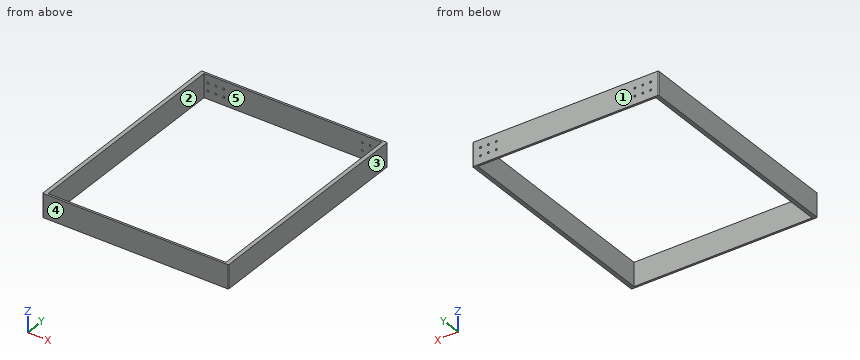
```python
from build123d import *

# Parameters (mm, degrees)
SKETCH1_W           = 599.44
SKETCH1_H           = 723.9
SKETCH1_W_2         = 574.04
SKETCH1_H_2         = 711.2
BOSS_EXTRUDE1_DEPTH = 76.2
CUT_EXTRUDE1_REACH  = 789.191
SKETCH2_R           = 3.175
FILLET1_R           = 2.54


with BuildPart() as part:
    # Sketch1 → Boss-Extrude1 (new body)
    with BuildSketch(Plane.XY):
        Rectangle(SKETCH1_W, SKETCH1_H)
        Rectangle(SKETCH1_W_2, SKETCH1_H_2, mode=Mode.SUBTRACT)
    extrude(amount=BOSS_EXTRUDE1_DEPTH)

    # Sketch2 → Cut-Extrude1 (cut, up to next)
    with BuildSketch(Plane(origin=(0, 361.95, 0), x_dir=(1, 0, 0), z_dir=(0, 1, 0)), mode=Mode.PRIVATE) as cut_extrude1_sk1:
        with Locations(Location((-274.32, -50.8, 0), (0, 0, 270))):
            Circle(SKETCH2_R)
    cut_extrude1_tool1 = extrude(cut_extrude1_sk1.sketch, amount=-CUT_EXTRUDE1_REACH, mode=Mode.PRIVATE) & part.part
    # Sketch2 → Cut-Extrude1 (cut, up to next)
    with BuildSketch(Plane(origin=(0, 361.95, 0), x_dir=(1, 0, 0), z_dir=(0, 1, 0)), mode=Mode.PRIVATE) as cut_extrude1_sk2:
        with Locations(Location((-274.32, -25.4, 0), (0, 0, 270))):
            Circle(SKETCH2_R)
    cut_extrude1_tool2 = extrude(cut_extrude1_sk2.sketch, amount=-CUT_EXTRUDE1_REACH, mode=Mode.PRIVATE) & part.part
    # Sketch2 → Cut-Extrude1 (cut, up to next)
    with BuildSketch(Plane(origin=(0, 361.95, 0), x_dir=(1, 0, 0), z_dir=(0, 1, 0)), mode=Mode.PRIVATE) as cut_extrude1_sk3:
        with Locations(Location((-248.92, -50.8, 0), (0, 0, 270))):
            Circle(SKETCH2_R)
    cut_extrude1_tool3 = extrude(cut_extrude1_sk3.sketch, amount=-CUT_EXTRUDE1_REACH, mode=Mode.PRIVATE) & part.part
    # Sketch2 → Cut-Extrude1 (cut, up to next)
    with BuildSketch(Plane(origin=(0, 361.95, 0), x_dir=(1, 0, 0), z_dir=(0, 1, 0)), mode=Mode.PRIVATE) as cut_extrude1_sk4:
        with Locations(Location((-248.92, -25.4, 0), (0, 0, 270))):
            Circle(SKETCH2_R)
    cut_extrude1_tool4 = extrude(cut_extrude1_sk4.sketch, amount=-CUT_EXTRUDE1_REACH, mode=Mode.PRIVATE) & part.part
    # Sketch2 → Cut-Extrude1 (cut, up to next)
    with BuildSketch(Plane(origin=(0, 361.95, 0), x_dir=(1, 0, 0), z_dir=(0, 1, 0)), mode=Mode.PRIVATE) as cut_extrude1_sk5:
        with Locations(Location((-223.52, -50.8, 0), (0, 0, 270))):
            Circle(SKETCH2_R)
    cut_extrude1_tool5 = extrude(cut_extrude1_sk5.sketch, amount=-CUT_EXTRUDE1_REACH, mode=Mode.PRIVATE) & part.part
    # Sketch2 → Cut-Extrude1 (cut, up to next)
    with BuildSketch(Plane(origin=(0, 361.95, 0), x_dir=(1, 0, 0), z_dir=(0, 1, 0)), mode=Mode.PRIVATE) as cut_extrude1_sk6:
        with Locations(Location((-223.52, -25.4, 0), (0, 0, 270))):
            Circle(SKETCH2_R)
    cut_extrude1_tool6 = extrude(cut_extrude1_sk6.sketch, amount=-CUT_EXTRUDE1_REACH, mode=Mode.PRIVATE) & part.part
    cut_extrude1_1 = cut_extrude1_tool1.solids().sort_by_distance((-274.32, 361.95, 50.8))[0]
    add(cut_extrude1_1, mode=Mode.SUBTRACT)
    cut_extrude1_2 = cut_extrude1_tool2.solids().sort_by_distance((-274.32, 361.95, 25.4))[0]
    add(cut_extrude1_2, mode=Mode.SUBTRACT)
    cut_extrude1_3 = cut_extrude1_tool3.solids().sort_by_distance((-248.92, 361.95, 50.8))[0]
    add(cut_extrude1_3, mode=Mode.SUBTRACT)
    cut_extrude1_4 = cut_extrude1_tool4.solids().sort_by_distance((-248.92, 361.95, 25.4))[0]
    add(cut_extrude1_4, mode=Mode.SUBTRACT)
    cut_extrude1_5 = cut_extrude1_tool5.solids().sort_by_distance((-223.52, 361.95, 50.8))[0]
    add(cut_extrude1_5, mode=Mode.SUBTRACT)
    cut_extrude1_6 = cut_extrude1_tool6.solids().sort_by_distance((-223.52, 361.95, 25.4))[0]
    add(cut_extrude1_6, mode=Mode.SUBTRACT)
    cut_extrude1 = cut_extrude1_1 + cut_extrude1_2 + cut_extrude1_3 + cut_extrude1_4 + cut_extrude1_5 + cut_extrude1_6  # Cut-Extrude1 as one shape, for the pattern or mirror that repeats it

    # Mirror1: Cut-Extrude1 across plane
    add(cut_extrude1.mirror(Plane(origin=(0, 0, 0), x_dir=(0, 0, 1), z_dir=(1, 0, 0))), mode=Mode.SUBTRACT)

    # Fillet1
    fillet1_edges = [part.edges().sort_by_distance(p)[0] for p in [
        (-299.72, -361.95, 38.1),
        (-299.72, 361.95, 38.1),
        (299.72, 361.95, 38.1),
        (299.72, -361.95, 38.1),
    ]]
    fillet(fillet1_edges, radius=FILLET1_R)


solid = part.part
```
Input: part model. Units: mm. Frame: model coordinates. Face numbers are marked on the shaded views. A direction names the side the tool comes from. Give positions to 0.01 mm unless a question says otherwise; leave off trailing zeros. Order: outer loops, then holes, each group sorted by start corner. A loop starts at its lowest first (then second) coordinate and runs counter-clockwise, first axis right, second up. Notation, with made-up numbers: M 65.5,-26 L 70.5,-26 A21 cw 70.5,3 Z; hole C 11.25,66.25 d11. An arc over 180 degrees is marked long. One line per question, with ' | ' between items.
1) Access query for the marked faces 1 and 2. Directions: +Z, -Z, +X, -X, +Y, -Y. A direction counts if a zero-diameter tool reaches every point of the face in a straight line with its end or side. Return the directions, or none.
Filled in:
face 1: +Z, -Z, +X, -X, +Y | face 2: +Z, -Z
2) Contact query for flat-ended pins moving along their axis: P1, Ø10, axis at x = -248.92, z = 50.8, coming from the +Y side; P2, Ø5, axis at x = 223.52, z = 25.4, coming from the +Y side. Output: stop coordinate, or through.
Filled in:
P1: stops at y = 361.95 | P2: stops at y = -355.6
3) Draft query along X for the marked faces 3, 4 and 5. Return one class per face: pulls with the +X half, pulls with the -X half, needs draft (parallel to the pull), parting line crosses it, or undercut.
Filled in:
face 3: pulls with the +X half | face 4: needs draft | face 5: undercut
4) Section C-C on z = 8. Output: boundary loops of the cut face in (x, y).
Filled in:
outline: M -299.72,-359.41 A2.54 ccw -297.18,-361.95 L 297.18,-361.95 A2.54 ccw 299.72,-359.41 L 299.72,359.41 A2.54 ccw 297.18,361.95 L -297.18,361.95 A2.54 ccw -299.72,359.41 Z; hole M -287.02,-355.6 L 287.02,-355.6 L 287.02,355.6 L -287.02,355.6 Z
5) Ray query, L1, parallel to Z at x = -223, y = 358; L2, parallel to Z at x = 274, y = 357; L3, parallel to X at y = -110, z = 65. Return the intervals inside material, ascending.
Filled in:
L1: z = 0 to 22.27, 28.53 to 47.67, 53.93 to 76.2 | L2: z = 0 to 22.24, 28.56 to 47.64, 53.96 to 76.2 | L3: x = -299.72 to -287.02, 287.02 to 299.72
6) Section A-A on y = 238.5. Output: boundary loops of the cut face in (x, z), and give its area (3 significant figures).
Filled in:
outline: M -299.72,0 L -287.02,0 L -287.02,76.2 L -299.72,76.2 Z; M 287.02,0 L 299.72,0 L 299.72,76.2 L 287.02,76.2 Z | area: 1,940 mm2
7) Section B-B on x = -138. Output: boundary loops of the cut face in (y, z).
Filled in:
outline: M -361.95,0 L -355.6,0 L -355.6,76.2 L -361.95,76.2 Z; M 355.6,0 L 361.95,0 L 361.95,76.2 L 355.6,76.2 Z
